from build123d import *

# Parameters (mm, degrees)
F0_R      = 2.5
F1_DEPTH  = 3.175
F2_R      = 1.75
F3_DEPTH  = 8.5
F4_SIZE   = 0.75
F5_R      = 1
F7_R      = 1.5
F9_R      = 1.5
F10_DEPTH = 1
F11_SIZE  = 0.99999


# Not quite as in the source:
# - a fillet or chamfer is up to 0.001 mm smaller than in the source, because OpenCascade refuses the exact size


with BuildPart() as f1:
    # F0 (on Top) → F1 (new body)
    with BuildSketch(Plane.XY):
        Circle(F0_R)
    extrude(amount=F1_DEPTH)

    # F2 (on face) → F3 (join)
    with BuildSketch(Plane.XY.offset(3.175)):
        Circle(F2_R)
    extrude(amount=F3_DEPTH)

    # F4
    f4_edges = [f1.edges().sort_by_distance(p)[0] for p in [
        (-1.75, 0, 11.675),
    ]]
    chamfer(f4_edges, length=F4_SIZE)

    # F5 (on face) → F8 section 0
    with BuildSketch(Plane.XY.offset(11.675)):
        Circle(F5_R)
    # F7 (on offset) → F8 section 1
    with BuildSketch(Plane.XY.offset(16.175)):
        Circle(F7_R)
    loft()

    # F9 (on face) → F10 (join)
    with BuildSketch(Plane.XY.offset(16.175)):
        Circle(F9_R)
    extrude(amount=F10_DEPTH)

    # F11 (size 1 in the source; OpenCascade refuses exactly that, so slightly less here)
    f11_edges = [f1.edges().sort_by_distance(p)[0] for p in [
        (-1.5, 0, 17.175),
    ]]
    chamfer(f11_edges, length=F11_SIZE)


solid = f1.part
The model under review builds one solid part; all positions refer to its coordinate system, in mm. A direction names the side the tool comes from. Coordinates: 2 decimals unless noted, no trailing zeros. Write each loop counter-clockwise with the first axis right and the second up, starting at its lowest first coordinate (ties: lowest second). Pieces come first, ordered by that corner, then holes. Notation, with made-up numbers: M 86,-13 L 117,-13 A21 cw 117,-1 Z; hole C -8.75,-17.75 d1. An arc over 180 degrees is marked long. Put each result on its own line as item: value.
1) Draft analysis for pull direction Z (two halves, no side actions). For faces 3 (the conical face through (1.16, -0.48, 13.96)), 4 (the flat face through (0, 0, 17.175)), 5 (the cylindrical face through (1.617, -0.67, 6.996)), state which applies: released by +Z, released by -Z, zero draft, split by the parting line, or undercut.
Computed:
face 3: undercut
face 4: released by +Z
face 5: zero draft
2) Add section D-D on x = 2.05. Give the boundary of the cut face in (y, z) (3 decimals).
Computed:
outline: M -1.431,0 L 1.431,0 L 1.431,3.175 L -1.431,3.175 Z
3) Add section B-B on y = -2. Give the boundary of the cut face in (x, z) (3 decimals), then the cut area to 4 significant figures.
Computed:
outline: M -1.5,0 L 1.5,0 L 1.5,3.175 L -1.5,3.175 Z
area: 9.525 mm2
4) Clearance check with flat-ended pins moving along their axes: pin 1 Ø2 at (x, z) = (1, 11) entering from +Y; pin 2 Ø1 at (x, y) = (1, 0.5) entering from +Z; pin 3 Ø1 at (x, z) = (0, 5.5) entering from -Y. State where each tip first meets the part, or that it passes through.
Computed:
pin 1: stops at y = 1.75
pin 2: stops at z = 17.06
pin 3: stops at y = -1.75
5) For faces 1 (the flat face through (-2, -1, 3.175)), 2 (the flat face through (0, 0, 0)), list the 3-axis set-ups (+Z, -Z, +X, -X, +Y, -Y) from which the entire face can be reached by the end or side of a thin tool; tool diameter is ignored.
Computed:
face 1: +Z
face 2: -Z, +X, -X, +Y, -Y
6) Wall thickness on probe 1 along Z at (x, y) = (1.15, 2) (3 decimals); probe 2 along Y at (x, z) = (-0.9, 5.5); probe 3 along X at (y, z) = (-0.1, 5.5): over which ranges is each line inside the solid? List them lowest first. Write a range as [from, to].
Computed:
probe 1: z = [0, 3.175]
probe 2: y = [-1.5, 1.5]
probe 3: x = [-1.75, 1.75]
7) Add section C-C on z = 1.5. Give the boundary of the cut face in (x, y).
Computed:
outline: C 0,0 d5
